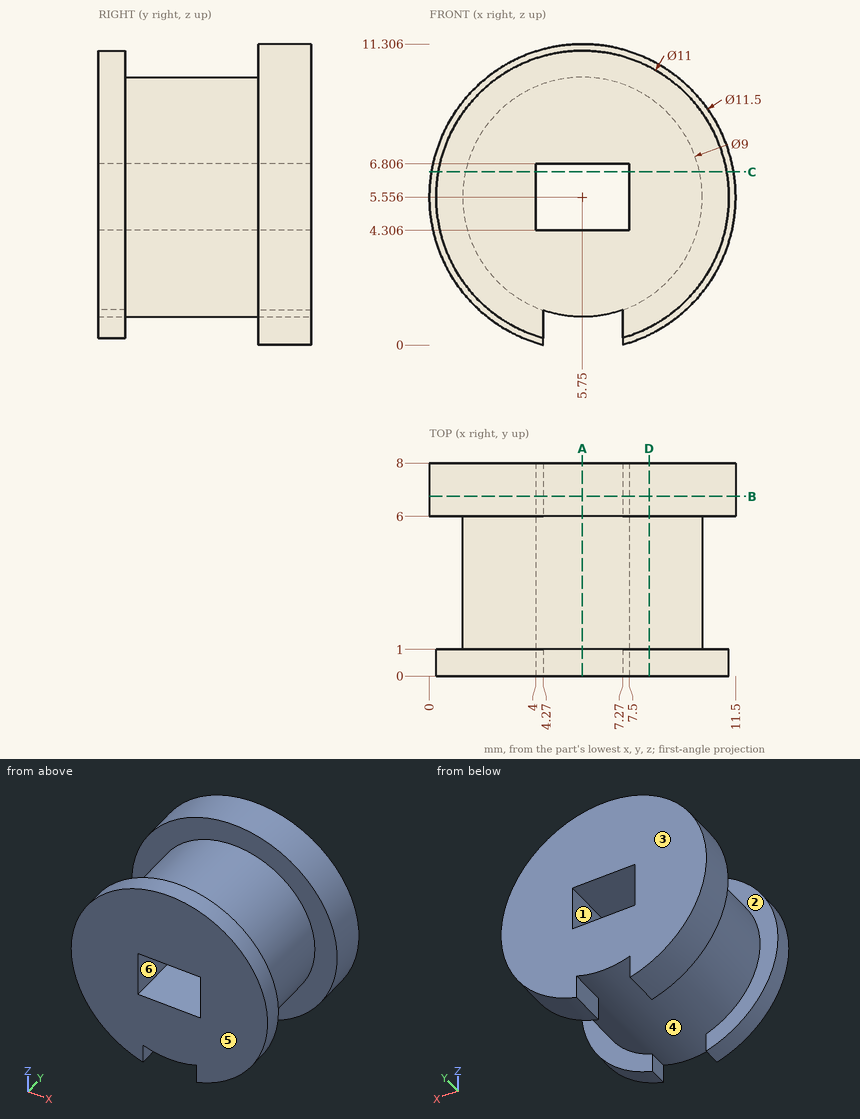
Here's the drawing with two shaded views (mm, measured from the low corner). I have some questions. A direction names the side the tool comes from. Give positions to 0.01 mm unless a question says otherwise; leave off trailing zeros. Order: outer loops, then holes, each group sorted by start corner. A loop starts at its lowest first (then second) coordinate and runs counter-clockwise, first axis right, second up. Notation, with made-up numbers: M -25.75,-2 L -1.75,-2 A22 ccw -1.75,5 Z; hole C -26.5,18 d3. An arc over 180 degrees is marked long. Answer as a JSON object with one key per item and string values. Group by question number.
1) I'm going to push flat-ended pins straight in: pin 1 Ø1 at (y, z) = (4.5, 4.5) entering from +X (1 decimal); pin 2 Ø1 at (x, y) = (6, 2.5) entering from -Z; pin 3 Ø2 at (x, y) = (4.5, 1.5) entering from +Z. Where does each tip first touch, or does it pass through?
2) Suppose I cut it at D-D, the plane x = 8.25. Write out the boundary of the cut face in (y, z) (1 decimal).
3) We'd pull the mould along Y, two halves only. Please class the marked faces 3, 4, 5 and 6: pulls with the +Y half, pulls with the -Y half, needs draft (parallel to the pull), parting line crosses it, or undercut.
4) Suppose I cut it at B-B, the plane y = 6.75. Write out the boundary of the cut face in (x, z), plus the area to 3 significant figures.
5) Please list where these lines run through material, in increasing order: L1, parallel to X at y = 1.5, z = 5.5; L2, parallel to X at y = 7.25, z = 5.75; L3, parallel to Y at x = 1.75, z = 7.75. Write a range as [from, to].
6) On a 3-axis mill with a long thin cutter (end or side, diameter ignored), from which of +Z, -Z, +X, -X, +Y, -Y can I reach the whole of each face in a straight line? I mean the marked faces 1 and 2. Say none if no direction works.
7) Suppose I cut it at C-C, the plane z = 6.5. Write out the boundary of the cut face in (x, y).
8) Suppose I cut it at A-A, the plane x = 5.75. Write out the boundary of the cut face in (y, z).
Results found:
{
 "1": {"pin 1": "x = 10.2", "pin 2": "z = 1.06", "pin 3": "z = 11.04"},
 "2": {"outline": "M 0,0.7 L 1,0.7 L 1,1.8 L 6,1.8 L 6,0.4 L 8,0.4 L 8,10.7 L 6,10.7 L 6,9.3 L 1,9.3 L 1,10.5 L 0,10.5 Z"},
 "3": {"face 3": "pulls with the +Y half", "face 4": "undercut", "face 5": "pulls with the -Y half", "face 6": "needs draft"},
 "4": {"outline": "M 4.27,0 L 4.27,1.31 A4.5 ccw 7.27,1.32 L 7.27,0.01 A5.75 ccw long Z; hole M 4,4.31 L 7.5,4.31 L 7.5,6.81 L 4,6.81 Z", "area": "91.3 mm²"},
 "5": {"L1": "[1.25, 4], [7.5, 10.25]", "L2": "[0, 4], [7.5, 11.5]", "L3": "[0, 1], [6, 8]"},
 "6": {"face 1": "+Y, -Y", "face 2": "none"},
 "7": {"outline": "M 0.08,6 L 1.35,6 L 1.35,1 L 0.33,1 L 0.33,0 L 4,0 L 4,8 L 0.08,8 Z; M 7.5,0 L 11.17,0 L 11.17,1 L 10.15,1 L 10.15,6 L 11.42,6 L 11.42,8 L 7.5,8 Z"},
 "8": {"outline": "M 0,1.06 L 8,1.06 L 8,4.31 L 0,4.31 Z; M 0,6.81 L 8,6.81 L 8,11.31 L 6,11.31 L 6,10.06 L 1,10.06 L 1,11.06 L 0,11.06 Z"}
}
